Job drawing, mm, ordinate dimensions from the low corner. One solid piece. A direction names the side the tool comes from. Give positions to 0.01 mm unless a question says otherwise; leave off trailing zeros. Loops run counter-clockwise (first coordinate to the right, second up) from the corner with the lowest first, then second, coordinate; pieces in that order, holes last. Notation, with made-up numbers: (-18.75, 57) - (-13.75, 57) arc R21 ccw to (-13.75, 69) - close; hole circle Ø6 at (77, 21.5). An arc over 180 degrees is marked (long way). Answer as CSV lines item,"result". Start each with the question number.
Item 1: Drill centre lines: L1, parallel to X at y = 42, z = 21.5; L2, parallel to X at y = 26.5, z = 3.5 (1 decimal); L3, parallel to X at y = 85.5, z = 58. Where is each one in solid material? Low to high. Write a range as from..to.
Item 2: Saw through at A-A on z = 34. Give the cut face in (x, y) (1 decimal).
Item 3: Pin check, flat tips, straight feed: pin 1 (23.5 mm diameter, centred on x = 114.5, y = 114, fed in from +Z); pin 2 (9 mm diameter, centred on x = 113.5, y = 18, fed in from +Z); pin 3 (12 mm diameter, centred on x = 65, y = 128, fed in from -Z). Stop position of each tip, or through.
Item 4: Saw through at B-B on z = 20.5. Give the cut face in (x, y) (1 decimal).
Item 5: Saw through at D-D on z = 70.5. Give the cut face in (x, y) (1 decimal), plus the area to 3 significant figures.
Item 6: Saw through at C-C on z = 60.5. Give the cut face in (x, y) (1 decimal), plus the area to 3 significant figures.
Item 7: Pull direction X, two halves, no side cores. Call the marked faces 6, 7, 8 and 9: pulls with the +X half, pulls with the -X half, needs draft (parallel to the pull), parting line crosses it, or undercut.
Item 8: Tool access for the marked faces 1, 2, 3, 4 and 5: list every direction of +Z, -Z, +X, -X, +Y, -Y with a clear straight run to the whole face (end or side of a thin tool).
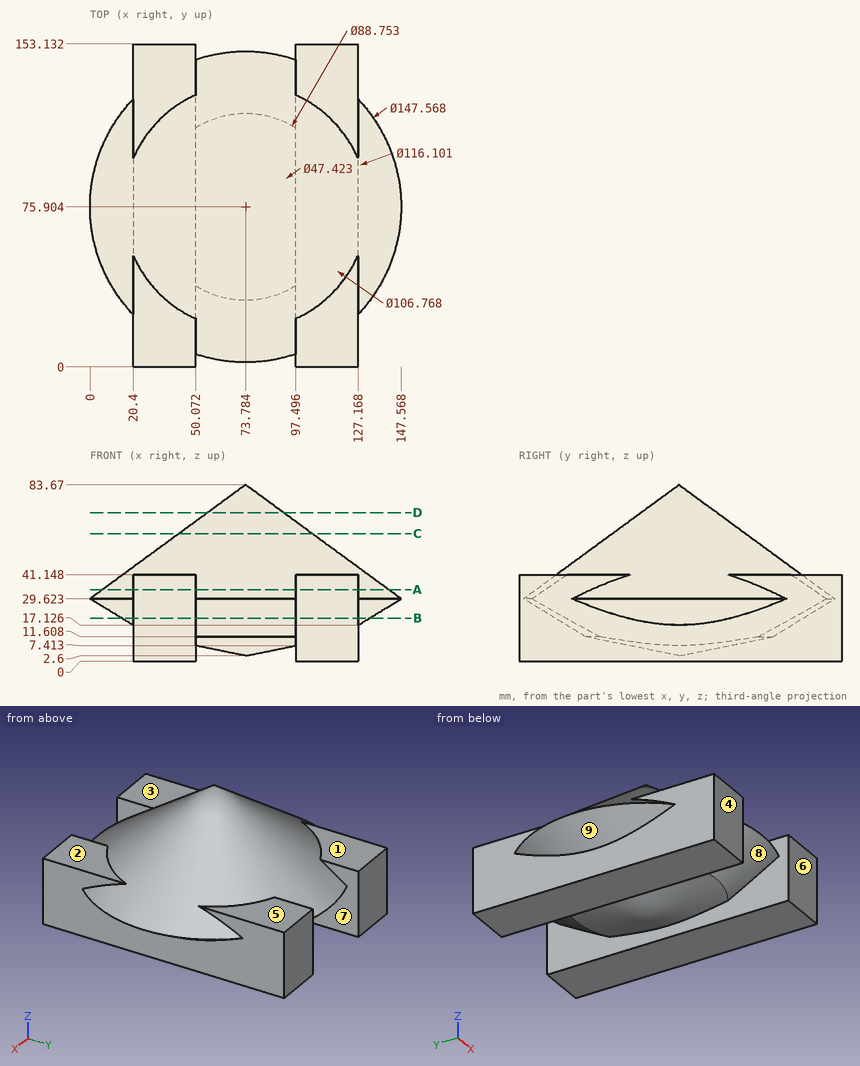
Responses:
1,L1,"20.4..127.17"
1,L2,"20.4..50.1, 97.5..127.2"
1,L3,"40.08..107.49"
2,outline,"(20.4, 0) - (50.1, 0) - (50.1, 12.4) arc R67.8 ccw to (97.5, 12.4) - (97.5, 0) - (127.2, 0) - (127.2, 34.1) arc R67.8 ccw to (127.2, 117.7) - (127.2, 153.1) - (97.5, 153.1) - (97.5, 139.4) arc R67.8 ccw to (50.1, 139.4) - (50.1, 153.1) - (20.4, 153.1) - (20.4, 117.7) arc R67.8 ccw to (20.4, 34.1) - close"
3,pin 1,"z = 51.43"
3,pin 2,"z = 41.15"
3,pin 3,"z = 13.11"
4,outline,"(20.4, 0) - (50.1, 0) - (50.1, 22) arc R58.9 ccw to (97.5, 22) - (97.5, 0) - (127.2, 0) - (127.2, 51) arc R58.9 ccw to (127.2, 100.8) - (127.2, 153.1) - (97.5, 153.1) - (97.5, 129.8) arc R58.9 ccw to (50.1, 129.8) - (50.1, 153.1) - (20.4, 153.1) - (20.4, 100.8) arc R58.9 ccw to (20.4, 51) - close"
5,outline,"circle Ø36 at (73.8, 75.9)"
5,area,"1,020 mm2"
6,outline,"circle Ø63.3 at (73.8, 75.9)"
6,area,"3,140 mm2"
7,face 6,"needs draft"
7,face 7,"undercut"
7,face 8,"undercut"
7,face 9,"pulls with the -X half"
8,face 1,"+Z, -X, +Y"
8,face 2,"+Z, +X, -Y"
8,face 3,"+Z, -X, -Y"
8,face 4,"+Z, -Z, +X, -X, -Y"
8,face 5,"+Z, +X, +Y"
